```python
from build123d import *

# Parameters (mm, degrees)
F1_DEPTH = 38.1
F0_W     = 31.75
F0_H     = 31.75
F2_DEPTH = 15.875
F3_DEPTH = 3.175


with BuildPart() as f1:
    # F0 (on Front) → F1 (new body, symmetric)
    with BuildSketch(Plane.XZ):
        Polygon((-38.1, -38.1), (38.1, -38.1), (38.1, -35.922859), (38.1, -4.172859), (38.1, 38.1), (26.53393, 38.1), (16.940894, 38.1), (-38.1, 38.1), align=None)
    extrude(amount=F1_DEPTH, both=True)

    # F0 (on Front) → F2 (join, symmetric)
    with BuildSketch(Plane.XZ):
        with Locations((53.975, -20.047859)):
            Rectangle(F0_W, F0_H)
    extrude(amount=F2_DEPTH, both=True)

    # F0 (on Front) → F3 (join, symmetric)
    with BuildSketch(Plane.XZ):
        Polygon((21.023035, 73.682681), (16.940894, 38.1), (26.53393, 38.1), align=None)
    extrude(amount=F3_DEPTH, both=True)


solid = f1.part
```
For this review, take the finished solid that the model builds, in its own axes (mm). A direction names the side the tool comes from. Coordinates: 2 decimals unless noted, no trailing zeros. Write each loop counter-clockwise with the first axis right and the second up, starting at its lowest first coordinate (ties: lowest second). Pieces come first, ordered by that corner, then holes. Notation, with made-up numbers: (81, 78) -> (101, 78) arc R31 ccw to (101, 107) -> close; hole circle Ø11 at (52, 66.25). An arc over 180 degrees is marked (long way). Put each result on its own line as item: value.
Q1. Clearance check with flat-ended pins moving along their axes: pin 1 Ø16 at (x, z) = (55.5, -16) entering from -Y (3 decimals); pin 2 Ø9.5 at (x, y) = (51, -4) entering from -Z; pin 3 Ø4 at (x, y) = (19.5, -24) entering from +Z. State where each tip first meets the part, or that it passes through.
From the geometry:
pin 1: stops at y = -15.875
pin 2: stops at z = -35.92
pin 3: stops at z = 38.1
Q2. Tool access review of faces 1 (the flat face through (22, 3.175, 48)), 2 (the flat face through (54, 0, -4.173)), 3 (the flat face through (54, 0, -35.923)), 4 (the flat face through (54, 15.875, -20)): name each direction out of +Z, -Z, +X, -X, +Y, -Y from which nothing blocks a thin tool from reaching the whole face with its end or side.
From the geometry:
face 1: +Z, +X, -X, +Y
face 2: +Z, +X, +Y, -Y
face 3: -Z, +X, +Y, -Y
face 4: +Z, -Z, +X, +Y
Q3. Take a section at C-C, the plane x = -8.5. State the section outline as (y, z) points.
From the geometry:
outline: (-38.1, -38.1) -> (38.1, -38.1) -> (38.1, 38.1) -> (-38.1, 38.1) -> close
Q4. Take a section at A-A, the plane y = -12. State the section outline as (x, z) points, then the cut area to 3 significant figures.
From the geometry:
outline: (-38.1, -38.1) -> (38.1, -38.1) -> (38.1, -35.92) -> (69.85, -35.92) -> (69.85, -4.17) -> (38.1, -4.17) -> (38.1, 38.1) -> (-38.1, 38.1) -> close
area: 6,810 mm2
Q5. Take a section at B-B, the plane z = -13. State the section outline as (x, y) points (3 decimals).
From the geometry:
outline: (-38.1, -38.1) -> (38.1, -38.1) -> (38.1, -15.875) -> (69.85, -15.875) -> (69.85, 15.875) -> (38.1, 15.875) -> (38.1, 38.1) -> (-38.1, 38.1) -> close
Q6. Wall thickness on L1, parallel to X at y = 28, z = 11; L2, parallel to Y at x = 50, z = -19 (3 decimals): over which ranges is each line inside the solid? List them lowest first.
From the geometry:
L1: x = -38.1 to 38.1
L2: y = -15.875 to 15.875
